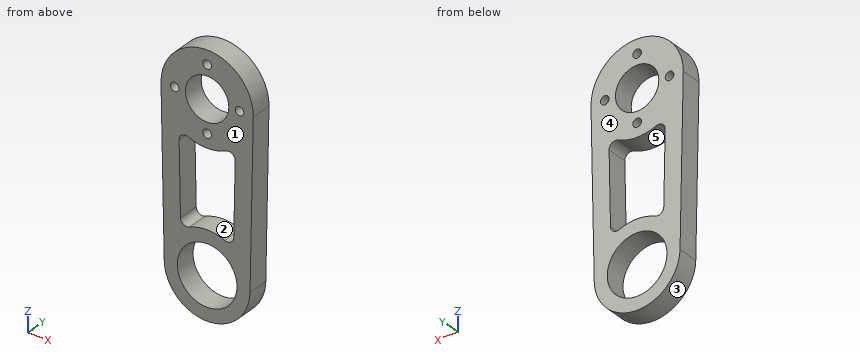
from build123d import *

# Parameters (mm, degrees)
SKETCH1_R           = 13.91353128
SKETCH1_R_2         = 2
SKETCH1_R_3         = 10.1
BOSS_EXTRUDE1_DEPTH = 10


with BuildPart() as part:
    # Sketch1 → Boss-Extrude1 (new body)
    with BuildSketch(Plane(origin=(0, 0, 0), x_dir=(1, 0, 0), z_dir=(0, 1, 0))):
        with BuildLine():
            Line((21.498983302, 0.209086062), (19.99622214, 77.513715994))
            ThreePointArc((19.99622214, 77.513715994), (0, 97.125), (-19.99622214, 77.513715994))
            Line((-19.99622214, 77.513715994), (-21.498983302, 0.209086062))
            ThreePointArc((-21.498983302, 0.209086062), (0, -21.5), (21.498983302, 0.209086062))
        make_face()
        with Locations(Location((0, 77.125, 0), (0, 0, 270))):
            Circle(SKETCH1_R, mode=Mode.SUBTRACT)
        with Locations(Location((0, 15.1, 0), (0, 0, 270))):
            Circle(SKETCH1_R_2, mode=Mode.SUBTRACT)
        with Locations(Location((15.1, 0, 0), (0, 0, 270))):
            Circle(SKETCH1_R_2, mode=Mode.SUBTRACT)
        with Locations(Location((0, -15.1, 0), (0, 0, 90))):
            Circle(SKETCH1_R_2, mode=Mode.SUBTRACT)
        with Locations(Location((0, 0, 0), (0, 0, 270))):
            Circle(SKETCH1_R_3, mode=Mode.SUBTRACT)
        with Locations(Location((-15.1, 0, 0), (0, 0, 90))):
            Circle(SKETCH1_R_2, mode=Mode.SUBTRACT)
        with BuildLine():
            Line((13.06692571, 22.394317415), (12.409386822, 56.196380392))
            ThreePointArc((12.409386822, 56.196380392), (11.016008446, 58.671921864), (8.182568929, 58.875463959))
            ThreePointArc((8.182568929, 58.875463959), (0, 57.125), (-8.182568929, 58.875463959))
            ThreePointArc((-8.182568929, 58.875463959), (-11.016008446, 58.671921864), (-12.409386822, 56.196380392))
            Line((-12.409386822, 56.196380392), (-13.06692571, 22.394317415))
            ThreePointArc((-13.06692571, 22.394317415), (-11.720069374, 19.832175089), (-8.834738892, 19.600953771))
            ThreePointArc((-8.834738892, 19.600953771), (0, 21.5), (8.834738892, 19.600953771))
            ThreePointArc((8.834738892, 19.600953771), (11.720069374, 19.832175089), (13.06692571, 22.394317415))
        make_face(mode=Mode.SUBTRACT)
    extrude(amount=BOSS_EXTRUDE1_DEPTH)


solid = part.part
Geometry: final body of the model. Coordinates: model frame, mm. Face numbers are marked on the shaded views. A direction names the side the tool comes from. Coordinates: 2 decimals unless noted, no trailing zeros. Order: outer loops, then holes, each group sorted by start corner. A loop starts at its lowest first (then second) coordinate and runs counter-clockwise, first axis right, second up.
(1) Access query for the marked faces 4 and 5. Directions: +Z, -Z, +X, -X, +Y, -Y. A direction counts if a zero-diameter tool reaches every point of the face in a straight line with its end or side. Return the directions, or none.
(2) Section query B-B (x = -7). Return the cut outline in (y, z), plus the area to 3 significant figures.
(3) Draft query along Z for the marked faces 1, 2 and 3. Return one class per face: pulls with the +Z half, pulls with the -Z half, needs draft (parallel to the pull), parting line crosses it, or undercut.
(4) Section query C-C (z = -90). Return the cut outline in (x, y).
(5) Section query D-D (x = 0). Return the cut outline in (y, z) (3 decimals).
(6) Section query A-A (y = 5.25). Return the cut outline in (x, z) (1 decimal).
(7) Material intervals for probe 1 along X at (y, z) = (6, 0); probe 2 along Z at (x, y) = (4.5, 5); probe 3 along Z at (x, y) = (-8, 2.5), sorted ascending.
(8) First-contact query: pin 1 (2.5 mm diameter, centred on x = 0, z = -15.1, fed in from -Y); pin 2 (1 mm diameter, centred on y = 2.5, z = -43, fed in from -X); pin 3 (1.5 mm diameter, centred on y = 8.5, z = -75.5, fed in from +X); pin 4 (3 mm diameter, centred on x = -12.5, y = 8.5, fed in from -Z). Flat tips, straight axial feed; report the tip coordinate or a pass-through.
Solution:
1. face 4: +Z, -Z, +X, -X, +Y
1. face 5: +Y, -Y
2. outline: (0, -95.86) - (10, -95.86) - (10, -89.15) - (0, -89.15) - close; (0, -65.1) - (10, -65.1) - (10, -58.39) - (0, -58.39) - close; (0, -20.33) - (10, -20.33) - (10, -7.28) - (0, -7.28) - close; (0, 7.28) - (10, 7.28) - (10, 20.33) - (0, 20.33) - close
2. area: 395 mm2
3. face 1: needs draft
3. face 2: undercut
3. face 3: pulls with the -Z half
4. outline: (-15.3, 0) - (-5.27, 0) - (-5.27, 10) - (-15.3, 10) - close; (5.27, 0) - (15.3, 0) - (15.3, 10) - (5.27, 10) - close
5. outline: (0, -97.125) - (10, -97.125) - (10, -91.039) - (0, -91.039) - close; (0, -63.211) - (10, -63.211) - (10, -57.125) - (0, -57.125) - close; (0, -21.5) - (10, -21.5) - (10, -17.1) - (0, -17.1) - close; (0, -13.1) - (10, -13.1) - (10, -10.1) - (0, -10.1) - close; (0, 10.1) - (10, 10.1) - (10, 13.1) - (0, 13.1) - close; (0, 17.1) - (10, 17.1) - (10, 21.5) - (0, 21.5) - close
6. outline: (-21.5, -0.2) - (-20, -77.5) arc R20 ccw to (20, -77.5) - (21.5, -0.2) arc R21.5 ccw (long way) to start; hole circle Ø4 at (-15.1, 0); hole circle Ø27.8 at (0, -77.1); hole (-13.1, -22.4) - (-12.4, -56.2) arc R3 ccw to (-8.2, -58.9) arc R20 cw to (8.2, -58.9) arc R3 ccw to (12.4, -56.2) - (13.1, -22.4) arc R3 ccw to (8.8, -19.6) arc R21.5 cw to (-8.8, -19.6) arc R3 ccw to start; hole circle Ø20.2 at (0, 0); hole circle Ø4 at (0, -15.1); hole circle Ø4 at (0, 15.1); hole circle Ø4 at (15.1, 0)
7. probe 1: x = -21.5 to -17.1, -13.1 to -10.1, 10.1 to 13.1, 17.1 to 21.5
7. probe 2: z = -96.61 to -90.29, -63.96 to -57.64, -21.02 to -9.04, 9.04 to 21.02
7. probe 3: z = -95.46 to -88.51, -65.74 to -58.79, -19.96 to -6.17, 6.17 to 19.96
8. pin 1: passes through
8. pin 2: stops at x = -20.68
8. pin 3: stops at x = 20.05
8. pin 4: stops at z = -93.83
